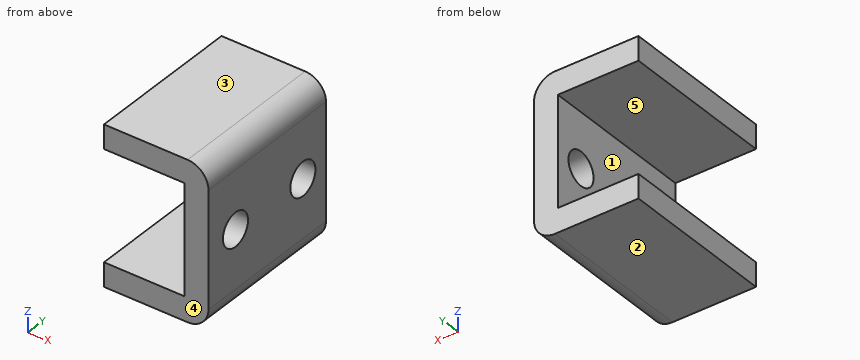
```python
from build123d import *

# Parameters (mm, degrees)
EXTRUDE_4_DEPTH     = 15
SKETCH_6_W          = 5.43
SKETCH_6_H          = 10.5
CUT_EXTRUDE_2_DEPTH = 15
SKETCH_7_W          = 2.285
SKETCH_7_H          = 10.5
CUT_EXTRUDE_3_DEPTH = 15
SKETCH_8_R          = 1.6
CUT_EXTRUDE_4_DEPTH = 10


with BuildPart() as part:
    # 草图1 → 凸台-拉伸4 (new body)
    with BuildSketch(Plane(origin=(0, 0, 0), x_dir=(1, 0, 0), z_dir=(0, 1, 0))):
        with BuildLine():
            Line((-35.94125392, 35.792894198), (-35.94125392, 20.722894198))
            Line((-35.94125392, 20.722894198), (-27.94125392, 20.722894198))
            ThreePointArc((-27.94125392, 20.722894198), (-26.527040358, 21.308680636), (-25.94125392, 22.722894198))
            Line((-25.94125392, 22.722894198), (-25.94125392, 33.792894198))
            ThreePointArc((-25.94125392, 33.792894198), (-26.527040358, 35.207107761), (-27.94125392, 35.792894198))
            Line((-27.94125392, 35.792894198), (-35.94125392, 35.792894198))
        make_face()
    extrude(amount=EXTRUDE_4_DEPTH)

    # 草图6 → 切除-拉伸2 (cut)
    with BuildSketch(Plane(origin=(0, 15, 0), x_dir=(1, 0, 0), z_dir=(0, 1, 0))):
        with Locations((-30.94125392, 28.257894198)):
            Rectangle(SKETCH_6_W, SKETCH_6_H)
    extrude(amount=-CUT_EXTRUDE_2_DEPTH, mode=Mode.SUBTRACT)

    # 草图7 → 切除-拉伸3 (cut)
    with BuildSketch(Plane(origin=(0, 15, 0), x_dir=(1, 0, 0), z_dir=(0, 1, 0))):
        with Locations((-34.79875392, 28.257894198)):
            Rectangle(SKETCH_7_W, SKETCH_7_H)
    extrude(amount=-CUT_EXTRUDE_3_DEPTH, mode=Mode.SUBTRACT)

    # 草图8 → 切除-拉伸4 (cut)
    with BuildSketch(Plane(origin=(-25.94125392, 0, 0), x_dir=(0, 0, -1), z_dir=(1, 0, 0))):
        with Locations((28.257894198, 12.049892986)):
            Circle(SKETCH_8_R)
        with Locations((28.257894198, 3.449892986)):
            Circle(SKETCH_8_R)
    extrude(amount=-CUT_EXTRUDE_4_DEPTH, mode=Mode.SUBTRACT)


solid = part.part
```
For this review, take the finished solid that the model builds, in its own axes (mm). Face numbers are marked on the shaded views. A direction names the side the tool comes from. Coordinates: 2 decimals unless noted, no trailing zeros. Order: outer loops, then holes, each group sorted by start corner. A loop starts at its lowest first (then second) coordinate and runs counter-clockwise, first axis right, second up. Notation, with made-up numbers: (33, -1.75) - (79, -1.75) arc R28 cw to (79, 29.25) - close; hole circle Ø8 at (31, 6). An arc over 180 degrees is marked (long way). Answer as a JSON object with one key per item and string values. Group by question number.
1. We need section C-C on z = -27. State the section outline as (x, y) points, then the cut area to 3 significant figures.
2. We need section B-B on y = 2.75. State the section outline as (x, z) points, then the cut area to 3 significant figures.
3. We need section A-A on x = -31.25. State the section outline as (y, z) points, then the cut area to 4 significant figures.
4. The part is to be moulded in two halves that separate along Z. For the marked faces 3, 4 and 5, say which applies: pulls with the +Z half, pulls with the -Z half, needs draft (parallel to the pull), parting line crosses it, or undercut.
5. Clearance check with flat-ended pins moving along their axes: P1, Ø3, axis at y = 10, z = -23.5, coming from the -X side; P2, Ø3.5, axis at y = 12.05, z = -28.26, coming from the -X side; P3, Ø5, axis at x = -31, z = -29, coming from the -Y side. State where each tip first meets the part, or that it passes through.
6. For the marked faces 1 and 2, list the 3-axis set-ups (+Z, -Z, +X, -X, +Y, -Y) from which the entire face can be reached by the end or side of a thin tool; tool diameter is ignored.
7. For probe 1 along Z at (x, y) = (-30.5, 8); probe 2 along X at (y, z) = (6, -31.5); probe 3 along Z at (x, y) = (-27, 8.75), list the stretches that pass through material, from the lowest coordinate up.
8. We need section D-D on y = 8. State the section outline as (x, z) points.
Final values:
{
 "1": {"outline": "(-28.23, 0) - (-25.94, 0) - (-25.94, 2.46) - (-28.23, 2.46) - close; (-28.23, 4.44) - (-25.94, 4.44) - (-25.94, 11.06) - (-28.23, 11.06) - close; (-28.23, 13.04) - (-25.94, 13.04) - (-25.94, 15) - (-28.23, 15) - close", "area": "25.2 mm²"},
 "2": {"outline": "(-35.94, -35.79) - (-27.94, -35.79) arc R2 ccw to (-25.94, -33.79) - (-25.94, -29.7) - (-28.23, -29.7) - (-28.23, -33.51) - (-35.94, -33.51) - close; (-35.94, -23.01) - (-28.23, -23.01) - (-28.23, -26.82) - (-25.94, -26.82) - (-25.94, -22.72) arc R2 ccw to (-27.94, -20.72) - (-35.94, -20.72) - close", "area": "61.4 mm²"},
 "3": {"outline": "(0, -35.79) - (15, -35.79) - (15, -33.51) - (0, -33.51) - close; (0, -23.01) - (15, -23.01) - (15, -20.72) - (0, -20.72) - close", "area": "68.55 mm²"},
 "4": {"face 3": "pulls with the +Z half", "face 4": "needs draft", "face 5": "undercut"},
 "5": {"P1": "x = -35.94", "P2": "x = -28.23", "P3": "through"},
 "6": {"face 1": "-X, +Y, -Y", "face 2": "-Z, +X, -X, +Y, -Y"},
 "7": {"probe 1": "-35.79 to -33.51, -23.01 to -20.72", "probe 2": "-28.23 to -25.94", "probe 3": "-35.56 to -20.96"},
 "8": {"outline": "(-35.94, -35.79) - (-27.94, -35.79) arc R2 ccw to (-25.94, -33.79) - (-25.94, -22.72) arc R2 ccw to (-27.94, -20.72) - (-35.94, -20.72) - (-35.94, -23.01) - (-28.23, -23.01) - (-28.23, -33.51) - (-35.94, -33.51) - close"}
}
